```python
from build123d import *

# Parameters (mm, degrees)
SKETCH1_R           = 1.5
BOSS_EXTRUDE1_DEPTH = 55
SKETCH2_W           = 4
SKETCH2_H           = 1.5
BOSS_EXTRUDE2_DEPTH = 5
SKETCH3_R           = 1
CUT_EXTRUDE1_DEPTH  = 3.25


with BuildPart() as part:
    # Sketch1 → Boss-Extrude1 (new body)
    with BuildSketch(Plane(origin=(0, 0, 0), x_dir=(1, 0, 0), z_dir=(0, 1, 0))):
        Circle(SKETCH1_R)
    extrude(amount=BOSS_EXTRUDE1_DEPTH)

    # Sketch2 → Boss-Extrude2 (add)
    with BuildSketch(Plane(origin=(0, 55, 0), x_dir=(1, 0, 0), z_dir=(0, 1, 0))):
        Rectangle(SKETCH2_W, SKETCH2_H)
    extrude(amount=BOSS_EXTRUDE2_DEPTH)

    # Sketch3 → Cut-Extrude1 (cut, through all)
    with BuildSketch(Plane(origin=(0, 0, -0.75), x_dir=(-1, 0, 0), z_dir=(0, 0, -1))):
        with Locations((0, 58)):
            Circle(SKETCH3_R)
    extrude(amount=-CUT_EXTRUDE1_DEPTH, mode=Mode.SUBTRACT)


solid = part.part
```
Geometry: final body of the model. Coordinates: model frame, mm. A direction names the side the tool comes from. Coordinates: 2 decimals unless noted, no trailing zeros. Loops run counter-clockwise (first coordinate to the right, second up) from the corner with the lowest first, then second, coordinate; pieces in that order, holes last. Notation, with made-up numbers: (89, 84.25) -> (134, 84.25) arc R25 cw to (134, 123.25) -> close; hole circle Ø7 at (66, 28.5). An arc over 180 degrees is marked (long way). Use a Markdown table: item, result. Add a question column.
(1) Section query A-A, the plane x = 0. Return loops of the section in (y, z), plus the area to 4 significant figures.
(2) Mould query, pull axis X, two halves, no side actions, for faces 5 (the flat face through (-2, 57, 0)), 6 (the flat face through (0, 60, 0)), 7 (the cylindrical face through (-0.54, 58.84, -0.01)). Classes: pulls with the +X half, pulls with the -X half, needs draft (parallel to the pull), parting line crosses it, or undercut.
(3) Section query C-C, the plane z = 0. Return loops of the section in (x, y), plus the area to 3 significant figures.
(4) Section query D-D, the plane y = 47. Return loops of the section in (x, z), plus the area to 3 significant figures.
(5) Section query B-B, the plane y = 58. Return loops of the section in (x, z).
(6) Line query: line 1 along Y through (x, z) = (0, 0.05); line 2 along Z through (x, y) = (-1.7, 56); line 3 along X through (y, z) = (30.5, 0.1). Output: solid intervals per line, ascending.
(7) Access query for faces 1 (the cylindrical face through (-1.5, 27.12, -0.07)), 2 (the flat face through (0, 0, 0)), 3 (the flat face through (-0.5, 56.9, 0.75)), 4 (the flat face through (-0.5, 56.9, -0.75)). Directions: +Z, -Z, +X, -X, +Y, -Y. A direction counts if a zero-diameter tool reaches every point of the face in a straight line with its end or side. Return the directions, or none.
(8) Pin query (flat end, axial travel): pin 1 Ø0.6 at (x, z) = (1.5, -0.5) entering from -Y; pin 2 Ø1.6 at (x, y) = (0, 58) entering from -Z. Return the tip coordinate at first contact, or that it passes through.
Answer:
| question | item | result |
|---|---|---|
| 1 | outline | (0, -1.5) -> (55, -1.5) -> (55, -0.75) -> (57, -0.75) -> (57, 0.75) -> (55, 0.75) -> (55, 1.5) -> (0, 1.5) -> close; (59, -0.75) -> (60, -0.75) -> (60, 0.75) -> (59, 0.75) -> close |
| 1 | area | 169.5 mm^2 |
| 2 | face 5 | pulls with the -X half |
| 2 | face 6 | needs draft |
| 2 | face 7 | undercut |
| 3 | outline | (-2, 55) -> (-1.5, 55) -> (-1.5, 0) -> (1.5, 0) -> (1.5, 55) -> (2, 55) -> (2, 60) -> (-2, 60) -> close; hole circle Ø2 at (0, 58) |
| 3 | area | 182 mm^2 |
| 4 | outline | circle Ø3 at (0, 0) |
| 4 | area | 7.07 mm^2 |
| 5 | outline | (-2, -0.75) -> (-1, -0.75) -> (-1, 0.75) -> (-2, 0.75) -> close; (1, -0.75) -> (2, -0.75) -> (2, 0.75) -> (1, 0.75) -> close |
| 6 | line 1 | y = 0 to 57, 59 to 60 |
| 6 | line 2 | z = -0.75 to 0.75 |
| 6 | line 3 | x = -1.5 to 1.5 |
| 7 | face 1 | -Y |
| 7 | face 2 | +Z, -Z, +X, -X, -Y |
| 7 | face 3 | +Z, +X, -X, +Y |
| 7 | face 4 | -Z, +X, -X, +Y |
| 8 | pin 1 | stops at y = 0 |
| 8 | pin 2 | passes through |
